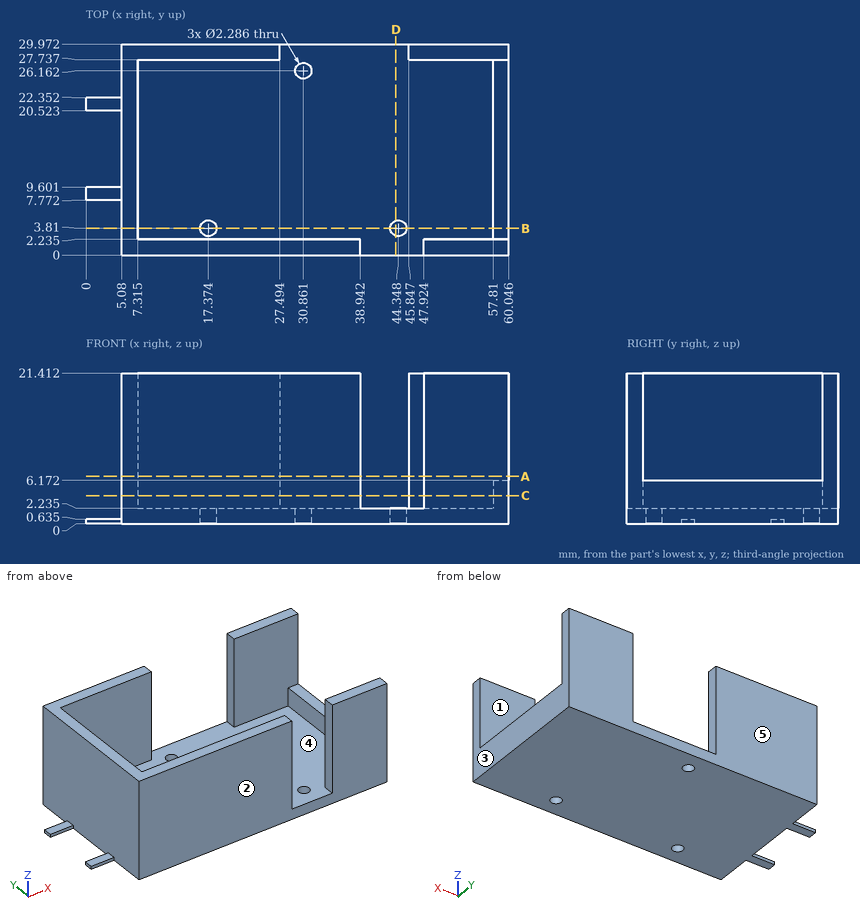
Geometry: see drawing. Coordinates: mm, zero at the bounding-box minimum. A direction names the side the tool comes from. Round coordinates to 2 decimals unless told otherwise and drop trailing zeros. Loops run counter-clockwise (first coordinate to the right, second up) from the corner with the lowest first, then second, coordinate; pieces in that order, holes last. Notation, with made-up numbers: (-30.5, 27) -> (7.5, 27) arc R26 ccw to (7.5, 65) -> close; hole circle Ø11 at (-4, 38.25). An arc over 180 degrees is marked (long way). One line per question, with ' | ' between items. Start each with the question number.
1. Mould query, pull axis X, two halves, no side actions, for the marked faces 3, 4 and 5. Classes: pulls with the +X half, pulls with the -X half, needs draft (parallel to the pull), parting line crosses it, or undercut.
2. Contact query for flat-ended pins moving along their axis: pin 1 (3 mm diameter, centred on x = 47.5, y = 7.5, fed in from +Z) (1 decimal); pin 2 (0.7 mm diameter, centred on x = 3, z = 0.5, fed in from -Y); pin 3 (1.1 mm diameter, centred on x = 59, y = 11, fed in from +Z). Output: stop coordinate, or through.
3. Section B-B on y = 3.81. Output: boundary loops of the cut face in (x, z) (1 decimal), and give its area (3 significant figures).
4. Line query: line 1 along X through (y, z) = (10, 3.5) (1 decimal); line 2 along Y through (x, z) = (14, 14) (1 decimal); line 3 along Z through (x, y) = (29.5, 22) (1 decimal). Output: solid intervals per line, ascending. Write a range as [from, to].
5. Section C-C on z = 4. Output: boundary loops of the cut face in (x, y) (1 decimal).
6. Section A-A on z = 6.75. Output: boundary loops of the cut face in (x, y) (1 decimal).
7. Set-up query: the marked faces 1 and 2. Return all of +Z, -Z, +X, -X, +Y, -Y with unobstructed straight access to the full face (end or side cutting, diameter ignored); none if empty.
8. Section D-D on x = 44. Output: boundary loops of the cut face in (y, z) (1 decimal).
Returned:
1) face 3: pulls with the +X half | face 4: undercut | face 5: needs draft
2) pin 1: stops at z = 2.2 | pin 2: stops at y = 7.77 | pin 3: stops at z = 6.17
3) outline: (5.1, 0) -> (16.2, 0) -> (16.2, 2.2) -> (7.3, 2.2) -> (7.3, 21.4) -> (5.1, 21.4) -> close; (18.5, 0) -> (43.2, 0) -> (43.2, 2.2) -> (18.5, 2.2) -> close; (45.5, 0) -> (60, 0) -> (60, 6.2) -> (57.8, 6.2) -> (57.8, 2.2) -> (45.5, 2.2) -> close | area: 164 mm2
4) line 1: x = [5.1, 7.3], [57.8, 60] | line 2: y = [0, 2.2], [27.7, 30] | line 3: z = [0, 2.2]
5) outline: (5.1, 0) -> (38.9, 0) -> (38.9, 2.2) -> (7.3, 2.2) -> (7.3, 27.7) -> (27.5, 27.7) -> (27.5, 30) -> (5.1, 30) -> close; (45.8, 27.7) -> (57.8, 27.7) -> (57.8, 2.2) -> (47.9, 2.2) -> (47.9, 0) -> (60, 0) -> (60, 30) -> (45.8, 30) -> close
6) outline: (5.1, 0) -> (38.9, 0) -> (38.9, 2.2) -> (7.3, 2.2) -> (7.3, 27.7) -> (27.5, 27.7) -> (27.5, 30) -> (5.1, 30) -> close; (45.8, 27.7) -> (60, 27.7) -> (60, 30) -> (45.8, 30) -> close; (47.9, 0) -> (60, 0) -> (60, 2.2) -> (47.9, 2.2) -> close
7) face 1: +Z | face 2: +Z, -Z, +X, -X, -Y
8) outline: (0, 0) -> (2.7, 0) -> (2.7, 2.2) -> (0, 2.2) -> close; (4.9, 0) -> (30, 0) -> (30, 2.2) -> (4.9, 2.2) -> close
